Model file for the job. Use its own axes, mm. A direction names the side the tool comes from. Coordinates: 2 decimals unless noted, no trailing zeros. Write each loop counter-clockwise with the first axis right and the second up, starting at its lowest first coordinate (ties: lowest second). Pieces come first, ordered by that corner, then holes.
Q1. Band-saw the part on A-A, the plane x = 125. Write the cut outline in (y, z), plus the area to 3 significant figures.
Q2. Drill centre lines: probe 1 along Y at (x, z) = (2.85, 0) (3 decimals); probe 2 along Y at (x, z) = (102.5, 0); probe 3 along Y at (x, z) = (60, -5.5). Where is each one in solid material? Low to high.
Q3. Which spindle directions (+Z, -Z, +X, -X, +Y, -Y) get a long thin tool onto all of the face, cutting with end or side? Do faces 4 (the flat face through (0, 0, 0)), 5 (the cylindrical face through (1.52, 7.81, -1.73)), 6 (the cylindrical face through (92.86, -2.4, 7.63)). Say none if no direction does.
Q4. Pin check, flat tips, straight feed: P1, Ø8, axis at x = 66.5, z = 1, coming from the -Y side; P2, Ø1.8, axis at y = 5.5, z = 0, coming from the -X side; P3, Ø1.5, axis at x = 114, z = -3.5, coming from the +Y side. Stop position of each tip, or through.
Q5. Pull direction X, two halves, no side cores. Call faces 1 (the flat face through (3, 8, 2)), 2 (the cylindrical face through (8.1, -3.2, 10)), 3 (the conical face through (21.124, -2.606, 8.276)): released by +X, released by -X, zero draft, split by the parting line, or undercut.
from build123d import *

# Parameters (mm, degrees)
R_P_TITION_CIRCULAIRE1_COUNT = 3
CONG_1_R                     = 10


with BuildPart() as part:
    # Esquisse1 → Révolution1 (revolve)
    with BuildSketch(Plane.XY, mode=Mode.PRIVATE) as r_volution1_sk:
        with BuildLine():
            Line((0, 0), (0, 8))
            Line((0, 8), (3, 8))
            Line((3, 8), (3, 10.5))
            Line((3, 10.5), (13, 10.5))
            Line((13, 10.5), (24.141100896, 8))
            Line((24.141100896, 8), (162.699264746, 8))
            ThreePointArc((162.699264746, 8), (173.906942241, 9.530417624), (180, 0))
            Line((180, 0), (0, 0))
        make_face()
    revolve(r_volution1_sk.sketch.rotate(Axis((-57.132155607, 0, 0), (1, 0, 0)), 90), axis=Axis((-57.132155607, 0, 0), (1, 0, 0)))

    # Esquisse4 → Trou taraudé M2.51 (revolve, cut)
    with BuildSketch(Plane.ZX.offset(5.5)):
        Polygon((0, 0), (0, 5.115882135), (1.025, 4.5), (1.025, 0.325), (1.35, 0), align=None)
    trou_taraud_m2_51 = revolve(axis=Axis((-6.35, 5.5, 0), (1, 0, 0)), mode=Mode.SUBTRACT)

    # Répétition circulaire1: Trou taraudé M2.51 ×3 about axis
    r_p_tition_circulaire1_axis = Axis((0, 0, 0), (1, 0, 0))
    for i in range(1, R_P_TITION_CIRCULAIRE1_COUNT):
        add(trou_taraud_m2_51.rotate(r_p_tition_circulaire1_axis, i * 360 / R_P_TITION_CIRCULAIRE1_COUNT), mode=Mode.SUBTRACT)

    # Congé1
    cong_1_edges = [part.edges().sort_by_distance(p)[0] for p in [
        (162.699264746, 0, -8),
    ]]
    fillet(cong_1_edges, radius=CONG_1_R)


solid = part.part
Answer sheet:
1. outline: circle Ø16 at (0, 0)
1. area: 201 mm2
2. probe 1: y = -8 to 4.475, 6.525 to 8
2. probe 2: y = -8 to 8
2. probe 3: y = -5.81 to 5.81
3. face 4: +Z, -Z, -X, +Y, -Y
3. face 5: -X
3. face 6: none
4. P1: stops at y = -8
4. P2: stops at x = 4.58
4. P3: stops at y = 7.51
5. face 1: released by -X
5. face 2: zero draft
5. face 3: undercut
